Geometry check sheet. Reference: the model listing, model coordinates, mm. A direction names the side the tool comes from. Coordinates: 2 decimals unless noted, no trailing zeros. Write each loop counter-clockwise with the first axis right and the second up, starting at its lowest first coordinate (ties: lowest second). Pieces come first, ordered by that corner, then holes. Notation, with made-up numbers: (-10, -22.5) -> (19, -22.5) arc R26 ccw to (19, -5.5) -> close; hole circle Ø4 at (56, -38.5). An arc over 180 degrees is marked (long way). Answer in a Markdown table with one row per item. Add a question column.
1. Mould release check, pull along Z, two halves, no side actions. Record for faces 1 (the cylindrical face through (5.563, -12.165, -13.267)), 2 (the flat face through (92, 0, 0)), 3 (the conical face through (82.8, 0.2, 0.2)): pulls with the +Z half, pulls with the -Z half, needs draft (parallel to the pull), parting line crosses it, or undercut.
2. Cross-section at B-B on x = 49. Record the cut outline in (y, z), and give its area (3 significant figures).
3. Scan lines: L1, parallel to X at y = 5, z = 14.5; L2, parallel to X at y = 11, z = -1; L3, parallel to X at y = 0.5, z = 2. Record each from-to range of solid material in increasing order. Write a range as from..to.
4. Set-up check for faces 4 (the flat face through (0, 0, 0)), 5 (the cylindrical face through (51.067, -3.755, 11.923)): record each of +Z, -Z, +X, -X, +Y, -Y from which the full face is reachable in a straight line by a thin tool's end or side.
5. Depth check by flat-ended pin: P1, Ø2, axis at x = 68.5, z = -7, coming from the +Y side; P2, Ø3, axis at x = 66, z = 6.5, coming from the -Y side; P3, Ø12, axis at x = 21, z = -8, coming from the -Y side. Enter the tip coordinate at first touch or a pass-through.
6. Cross-section at A-A on y = 0. Record the cut outline in (x, z) (1 decimal), and give its area (3 significant figures).
```python
from build123d import *

# Parameters (mm, degrees)
CHAMFER1_SIZE = 1


with BuildPart() as part:
    # Sketch1 → Revolve1 (revolve)
    with BuildSketch(Plane.XY, mode=Mode.PRIVATE) as revolve1_sk:
        Polygon((0, 0), (0, 18), (10, 18), (10, 12.5), (92, 12.5), (92, 0), align=None)
    revolve(revolve1_sk.sketch.rotate(Axis((0, 0, 0), (1, 0, 0)), 90), axis=Axis((0, 0, 0), (1, 0, 0)))

    # Sketch2 → Cut-Revolve1 (revolve, cut)
    with BuildSketch(Plane.XY, mode=Mode.PRIVATE) as cut_revolve1_sk:
        Polygon((83, -12.5), (82.625, 12.5), (80.5, 12.5), (80.5, -12.5), align=None)
    revolve(cut_revolve1_sk.sketch.rotate(Axis((80.5, 12.5, 0), (0, -1, 0)), 227.113167314), axis=Axis((80.5, 12.5, 0), (0, -1, 0)), mode=Mode.SUBTRACT)

    # Chamfer1
    chamfer1_edges = [part.edges().sort_by_distance(p)[0] for p in [
        (92, 0, -12.5),
        (0, 0, -18),
    ]]
    chamfer(chamfer1_edges, length=CHAMFER1_SIZE)


solid = part.part
```
Results found:
| question | item | result |
|---|---|---|
| 1 | face 1 | parting line crosses it |
| 1 | face 2 | needs draft |
| 1 | face 3 | undercut |
| 2 | outline | circle Ø25 at (0, 0) |
| 2 | area | 491 mm^2 |
| 3 | L1 | x = 0..10 |
| 3 | L2 | x = 0..78.6, 82.4..92 |
| 3 | L3 | x = 0..79.35, 81.65..92 |
| 4 | face 4 | +Z, -Z, -X, +Y, -Y |
| 4 | face 5 | +X |
| 5 | P1 | stops at y = 10.97 |
| 5 | P2 | stops at y = -11.46 |
| 5 | P3 | stops at y = -12.34 |
| 6 | outline | (0, -17) -> (1, -18) -> (10, -18) -> (10, -12.5) -> (91, -12.5) -> (92, -11.5) -> (92, 11.5) -> (91, 12.5) -> (10, 12.5) -> (10, 18) -> (1, 18) -> (0, 17) -> close; hole circle Ø4.6 at (80.5, 0) |
| 6 | area | 2,390 mm^2 |
